from build123d import *

# Parameters (mm, degrees)
SKETCH1_W           = 30
SKETCH1_H           = 30
BOSS_EXTRUDE2_DEPTH = 2
SKETCH1_6_W         = 34
SKETCH1_6_H         = 34
SKETCH1_6_W_2       = 30
SKETCH1_6_H_2       = 30
BOSS_EXTRUDE3_DEPTH = 5
FILLET1_R           = 1.5
SKETCH2_R           = 0.9
BOSS_EXTRUDE4_DEPTH = 1


with BuildPart() as part:
    # Sketch1 → Boss-Extrude2 (new body)
    with BuildSketch(Plane(origin=(0, 0, 0), x_dir=(1, 0, 0), z_dir=(0, 1, 0))):
        Rectangle(SKETCH1_W, SKETCH1_H)
    extrude(amount=BOSS_EXTRUDE2_DEPTH)

    # Sketch1<6> → Boss-Extrude3 (add)
    with BuildSketch(Plane(origin=(0, 0, 0), x_dir=(1, 0, 0), z_dir=(0, 1, 0))):
        Rectangle(SKETCH1_6_W, SKETCH1_6_H)
        Rectangle(SKETCH1_6_W_2, SKETCH1_6_H_2, mode=Mode.SUBTRACT)
    extrude(amount=BOSS_EXTRUDE3_DEPTH)

    # Fillet1
    fillet1_edges = [part.edges().sort_by_distance(p)[0] for p in [
        (15, 3.5, -15),
        (-15, 3.5, -15),
        (-15, 3.5, 15),
        (15, 3.5, 15),
    ]]
    fillet(fillet1_edges, radius=FILLET1_R)

    # Sketch2 → Boss-Extrude4 (add)
    with BuildSketch(Plane(origin=(0, 5, 0), x_dir=(1, 0, 0), z_dir=(0, 1, 0))):
        with Locations((0, 16)):
            Circle(SKETCH2_R)
        with Locations((2.5, 16)):
            Circle(SKETCH2_R)
        with Locations((-2.5, 16)):
            Circle(SKETCH2_R)
    extrude(amount=BOSS_EXTRUDE4_DEPTH)


solid = part.part
Input: part model. Units: mm. Frame: model coordinates. A direction names the side the tool comes from. Give positions to 0.01 mm unless a question says otherwise; leave off trailing zeros. Order: outer loops, then holes, each group sorted by start corner. A loop starts at its lowest first (then second) coordinate and runs counter-clockwise, first axis right, second up.
Q1. Section B-B on y = 3.05. Output: boundary loops of the cut face in (x, z).
Checked values:
outline: (-17, -17) - (17, -17) - (17, 17) - (-17, 17) - close; hole (-15, -13.5) arc R1.5 ccw to (-13.5, -15) - (13.5, -15) arc R1.5 ccw to (15, -13.5) - (15, 13.5) arc R1.5 ccw to (13.5, 15) - (-13.5, 15) arc R1.5 ccw to (-15, 13.5) - close
Q2. Ray query, probe 1 along Z at (x, y) = (-11, 4.75); probe 2 along Y at (x, z) = (-10, 13.5). Return the intervals inside material, ascending.
Checked values:
probe 1: z = -17 to -15, 15 to 17
probe 2: y = 0 to 2
Q3. Set-up query: faces 1 (the flat face through (0, 2, -17)), 2 (the cylindrical face through (2.38, 5.49, -16.89)). Return all of +Z, -Z, +X, -X, +Y, -Y with unobstructed straight access to the full face (end or side cutting, diameter ignored); none if empty.
Checked values:
face 1: -Z, +X, -X, +Y, -Y
face 2: +Y
Q4. Draft query along X for faces 3 (the flat face through (2, 6, -16)), 4 (the flat face through (17, 2, 0)), 5 (the flat face through (-17, 2, 0)), 6 (the cylindrical face through (-2.62, 5.49, -16.89)). Return one class per face: +X half, -X half, draft (parallel to the pull), parting line (faces both ways), or undercut.
Checked values:
face 3: draft
face 4: +X half
face 5: -X half
face 6: undercut
Q5. Section C-C on z = -12. Output: boundary loops of the cut face in (x, y).
Checked values:
outline: (-17, 0) - (17, 0) - (17, 5) - (15, 5) - (15, 2) - (-15, 2) - (-15, 5) - (-17, 5) - close
Q6. Section A-A on x = 4. Output: boundary loops of the cut face in (y, z).
Checked values:
outline: (0, -17) - (5, -17) - (5, -15) - (2, -15) - (2, 15) - (5, 15) - (5, 17) - (0, 17) - close
Q7. Contact query for a flat-ended pin moving along its axis: pin 1 Ø10 at (x, z) = (-8.5, -8) entering from +Y. Output: stop coordinate, or through.
Checked values:
pin 1: stops at y = 2
Q8. Section D-D on y = 5.45. Output: boundary loops of the cut face in (x, z), and give its area (3 significant figures).
Checked values:
outline: circle Ø1.8 at (-2.5, -16); circle Ø1.8 at (0, -16); circle Ø1.8 at (2.5, -16)
area: 7.63 mm2
